Source: CAD feature listing. Evaluate the final solid. Frame: model axes, mm. A direction names the side the tool comes from. Give positions to 0.01 mm unless a question says otherwise; leave off trailing zeros. Order: outer loops, then holes, each group sorted by start corner. A loop starts at its lowest first (then second) coordinate and runs counter-clockwise, first axis right, second up. Notation, with made-up numbers: (75.5, 55.25) - (100.5, 55.25) arc R19 cw to (100.5, 80.25) - close; hole circle Ø8 at (56.5, 52). An arc over 180 degrees is marked (long way). Write each question's results on one line, items separated by ' | '. Start each with the question number.
Item 1: Section A-A on z = 0. Output: boundary loops of the cut face in (x, y).
Item 2: Section C-C on z = 9.5. Output: boundary loops of the cut face in (x, y).
Item 3: Set-up query: faces 1 (the cylindrical face through (14.21, -1.76, 13.3)), 2 (the cylindrical face through (-5.106, -1.765, 22.393)), 3 (the cylindrical face through (14.21, -1.76, -13.3)). Return all of +Z, -Z, +X, -X, +Y, -Y with unobstructed straight access to the full face (end or side cutting, diameter ignored); none if empty.
Item 4: Line query: line 1 along X through (y, z) = (-7.5, 17.7); line 2 along Z through (x, y) = (9.5, -8); line 3 along X through (y, z) = (-3.5, -0.5). Output: solid intervals per line, ascending.
Item 5: Contact query for flat-ended pins moving along their axis: pin 1 Ø5.5 at (x, z) = (0, 9.5) entering from -Y; pin 2 Ø3 at (x, z) = (-9.5, 0) entering from +Y; pin 3 Ø5.5 at (x, z) = (6, -15.5) entering from +Y; pin 4 Ø3.5 at (x, z) = (10, 15) entering from +Y. Output: stop coordinate, or through.
Item 6: Section D-D on y = -7. State how many separate pieces and enclosed holes the cut face has, and give its area (3 significant figures).
Item 7: Section B-B on x = 0. Output: boundary loops of the cut face in (y, z).
Item 8: Mould query, pull axis X, two halves, no side actions, for faces 4 (the cylindrical face through (5.1, -1.76, 22.41)), 5 (the cylindrical face through (-13.07, -6.83, -21.2)), 6 (the cylindrical face through (-14.21, -1.76, -13.3)). Classes: released by +X, released by -X, zero draft, split by the parting line, or undercut.
```python
from build123d import *

# Parameters (mm, degrees)
SKETCH1_W                                       = 29
SKETCH1_H                                       = 45.4
BOSS_EXTRUDE1_DEPTH                             = 10
CBORE_FOR_M5_HEX_HEAD_BOLT1_D                   = 5.5
CBORE_FOR_M5_HEX_HEAD_BOLT1_DEPTH               = 15
CBORE_FOR_M5_HEX_HEAD_BOLT1_CBORE_D             = 12.24
CBORE_FOR_M5_HEX_HEAD_BOLT1_CBORE_DEPTH         = 3.58
CBORE_FOR_M5_HEX_HEAD_BOLT1_TIP                 = 1.652366702
CSK_FOR_M3_FLAT_HEAD_MACHINE_SCREW1_D           = 3.4
CSK_FOR_M3_FLAT_HEAD_MACHINE_SCREW1_CSINK_D     = 6.3
CSK_FOR_M3_FLAT_HEAD_MACHINE_SCREW1_CSINK_ANGLE = 90
FILLET1_R                                       = 5
FILLET2_R                                       = 0.5


with BuildPart() as part:
    # Sketch1 → Boss-Extrude1 (new body)
    with BuildSketch(Plane(origin=(0, 0, 0), x_dir=(1, 0, 0), z_dir=(0, 1, 0))):
        Rectangle(SKETCH1_W, SKETCH1_H)
    extrude(amount=-BOSS_EXTRUDE1_DEPTH)

    # CBORE for M5 Hex Head Bolt1
    with Locations(Plane(origin=(0, 0, 0), x_dir=(1, 0, 0), z_dir=(0, 1, 0))):
        with Locations((-9.5, 17.7), (9.5, 17.7), (9.5, -17.7), (-9.5, -17.7)):
            CounterBoreHole(CBORE_FOR_M5_HEX_HEAD_BOLT1_D / 2, CBORE_FOR_M5_HEX_HEAD_BOLT1_CBORE_D / 2, CBORE_FOR_M5_HEX_HEAD_BOLT1_CBORE_DEPTH, depth=CBORE_FOR_M5_HEX_HEAD_BOLT1_DEPTH)
            with Locations((0, 0, -(CBORE_FOR_M5_HEX_HEAD_BOLT1_DEPTH + CBORE_FOR_M5_HEX_HEAD_BOLT1_TIP / 2))):  # 118° drill point
                Cone(0, CBORE_FOR_M5_HEX_HEAD_BOLT1_D / 2, CBORE_FOR_M5_HEX_HEAD_BOLT1_TIP, mode=Mode.SUBTRACT)

    # CSK for M3 Flat Head Machine Screw1 (through all)
    with Locations(Plane(origin=(0, -10, 0), x_dir=(-1, 0, 0), z_dir=(0, -1, 0))):
        with Locations((-9.5, 0), (0, 9.5), (9.5, 0), (0, -9.5)):
            CounterSinkHole(CSK_FOR_M3_FLAT_HEAD_MACHINE_SCREW1_D / 2, CSK_FOR_M3_FLAT_HEAD_MACHINE_SCREW1_CSINK_D / 2, counter_sink_angle=CSK_FOR_M3_FLAT_HEAD_MACHINE_SCREW1_CSINK_ANGLE)

    # Fillet1
    fillet1_edges = [part.edges().sort_by_distance(p)[0] for p in [
        (-14.5, -5, -22.7),
        (14.5, -5, -22.7),
        (14.5, -5, 22.7),
        (-14.5, -5, 22.7),
    ]]
    fillet(fillet1_edges, radius=FILLET1_R)

    # Fillet2
    fillet2_edges = [part.edges().sort_by_distance(p)[0] for p in [
        (-5.9709208, -1.79, 22.7),
        (-14.5, -1.79, 14.1709208),
        (14.5, -1.79, 14.1709208),
        (5.9709208, -1.79, 22.7),
        (14.5, -1.79, -14.1709208),
        (5.9709208, -1.79, -22.7),
        (-5.9709208, -1.79, -22.7),
        (-14.5, -1.79, -14.1709208),
    ]]
    fillet(fillet2_edges, radius=FILLET2_R)


solid = part.part
```
Evaluation:
1) outline: (-14.5, -10) - (-12.65, -10) - (-11.2, -8.55) - (-11.2, 0) - (-14.5, 0) - close; (-7.8, -8.55) - (-6.35, -10) - (6.35, -10) - (7.8, -8.55) - (7.8, 0) - (-7.8, 0) - close; (11.2, -8.55) - (12.65, -10) - (14.5, -10) - (14.5, 0) - (11.2, 0) - close
2) outline: (-14.5, -10) - (-3.15, -10) - (-1.7, -8.55) - (-1.7, 0) - (-14.5, 0) - close; (1.7, -8.55) - (3.15, -10) - (14.5, -10) - (14.5, 0) - (1.7, 0) - close
3) face 1: +Z, +Y | face 2: -X, +Y | face 3: -Z, +Y
4) line 1: x = -14.5 to -12.25, -6.75 to 6.75, 12.25 to 14.5 | line 2: z = -22.7 to -20.45, -14.95 to -1.7, 1.7 to 14.95, 20.45 to 22.7 | line 3: x = -14.5 to -11.12, -7.88 to 7.88, 11.12 to 14.5
5) pin 1: stops at y = -9.6 | pin 2: passes through | pin 3: stops at y = 0 | pin 4: stops at y = -3.58
6) separate pieces: 1 | enclosed holes: 8 | area: 1,160 mm^2
7) outline: (-10, -22.7) - (0, -22.7) - (0, -11.2) - (-8.55, -11.2) - (-10, -12.65) - close; (-10, -6.35) - (-8.55, -7.8) - (0, -7.8) - (0, 7.8) - (-8.55, 7.8) - (-10, 6.35) - close; (-10, 12.65) - (-8.55, 11.2) - (0, 11.2) - (0, 22.7) - (-10, 22.7) - close
8) face 4: released by +X | face 5: released by -X | face 6: undercut
